from build123d import *

# Parameters (mm, degrees)
F0_R     = 1.651
F1_DEPTH = 25.4
F4_W     = 3.124762
F4_H     = 1.046538
F5_DEPTH = 12.7


with BuildPart() as f1:
    # F0 (on Front) → F1 (new body)
    with BuildSketch(Plane.XZ):
        Circle(F0_R)
    extrude(amount=F1_DEPTH)

    # F2 (on Right) → F3 (revolve)
    with BuildSketch(Plane.YZ):
        with BuildLine():
            Line((0, 2.909936), (0, 0))
            Line((0, 0), (3.175, 0))
            ThreePointArc((3.175, 0), (2.340641, 2.145233), (0.276087, 3.162973))
            ThreePointArc((0.276087, 3.162973), (0.082381, 3.097187), (0, 2.909936))
        make_face()
    revolve(axis=Axis((0, 1.5875, 0), (0, 1, 0)))

    # F4 (on Right) → F5 (cut, symmetric)
    with BuildSketch(Plane.YZ):
        with Locations((2.691957, 0)):
            Rectangle(F4_W, F4_H)
    extrude(amount=F5_DEPTH, both=True, mode=Mode.SUBTRACT)


solid = f1.part
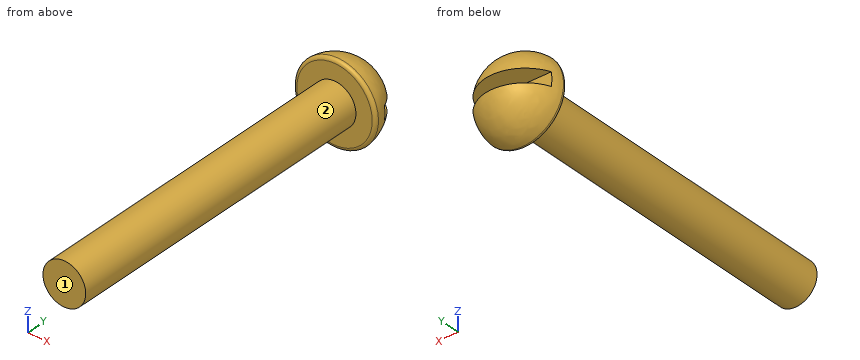
Part model, mm, in its own coordinate system. Face numbers are marked on the shaded views. A direction names the side the tool comes from. Coordinates: 2 decimals unless noted, no trailing zeros. Write each loop counter-clockwise with the first axis right and the second up, starting at its lowest first coordinate (ties: lowest second). Pieces come first, ordered by that corner, then holes. Notation, with made-up numbers: M 46.5,17 L 78.5,17 A26 ccw 78.5,48 Z; hole C -27.5,-23.5 d8. An arc over 180 degrees is marked long. Return JSON: item names as keys, results as strings.
1. Saw through at A-A, the plane y = -4.25. Write the cut outline in (x, z), then the cut area to 3 significant figures.
Determined:
{"outline": "C 0,0 d3.3", "area": "8.56 mm²"}
2. 3-axis set-ups, long thin cutter, end or side, ignore diameter. For the marked faces 1 and 2: which of +Z, -Z, +X, -X, +Y, -Y reach the whole face in a straight line?
Determined:
{"face 1": "+Z, -Z, +X, -X, -Y", "face 2": "-Y"}
3. Flat gauge pins, fed straight in: pin 1 Ø1.6 at (x, y) = (1, 1.5) entering from +Z; pin 2 Ø1.6 at (x, y) = (-0.5, 2.5) entering from -Z; pin 3 Ø2 at (y, z) = (-0.5, -2) entering from -X. Where does each tip first touch, or does it go through?
Determined:
{"pin 1": "z = 3.01", "pin 2": "z = -2.65", "pin 3": "x = -2.89"}
4. Probe L1, parallel to Z at x = 0, y = -9.5; L2, parallel to Y at x = 1, z = -0.25; L3, parallel to Y at x = -2.25, z = 0. List the from-to ranges inside material, lowest first.
Determined:
{"L1": "-1.65 to 1.65", "L2": "-25.4 to 1.13", "L3": "0 to 1.13"}
